Autodesk Inventor part; units mm, degrees
ref_plane "YZ Plane" through (0, 0, 0) normal (1, 0, 0) x (0, 1, 0)
ref_plane "XZ Plane" through (0, 0, 0) normal (0, 1, 0) x (-1, 0, 0)
ref_plane "XY Plane" through (0, 0, 0) normal (0, 0, 1) x (1, 0, 0)
sketch "Szkic2" plane through (0, 0, 0) normal (0, 1, 0) x (-1, 0, 0)
  line L0 (42.5, 23) -> (-42.5, 23)
  line L1 (-42.5, 23) -> (-42.5, -23)
  line L2 (-42.5, -23) -> (42.5, -23)
  line L3 (42.5, -23) -> (42.5, 23)
  line L4 (0, 91.0722) -> (0, -100.1143)
  line L5 (-78.4738, 0) -> (170.7955, 0)
  circle A0 centre (37.932, 17.8265) radius 2.25
  circle A1 centre (37.932, -17.8265) radius 2.25
  circle A2 centre (-37.932, 17.8265) radius 2.25
  circle A3 centre (-37.932, -17.8265) radius 2.25
  point P0 (0, 0)
  dimension "d7" = 46
  dimension "d8" = 85
  dimension "d14" = 4.5
  dimension "d16" = 35.653
  dimension "d18" = 23
  dimension "d21" = 75.864
  dimension "d22" = 42.5
extrude "Wyciągnięcie proste2" add sketch "Szkic2" along normal blind 2
sketch "Szkic3" plane through (0, 2, 0) normal (0, 1, 0) x (1, 0, 0)
  line L0 (-42.5, -23) -> (42.5, -23)
  line L1 (42.5, -23) -> (42.5, 23)
  line L2 (41.3, -23) -> (42.5, -23)
  line L3 (42.5, -23) -> (42.5, 23)
  line L4 (42.5, 23) -> (41.3, 23)
  line L5 (41.3, 23) -> (41.3, -23)
  line L6 (-42.5, 23) -> (-42.5, -23)
  line L7 (42.5, -23) -> (-42.5, -23)
  line L8 (-42.5, -23) -> (-42.5, -21.8)
  line L9 (-42.5, -21.8) -> (42.5, -21.8)
  line L10 (42.5, -21.8) -> (42.5, -23)
  line L11 (42.5, 23) -> (-42.5, 23)
  line L12 (-42.5, 23) -> (-42.5, 21.8)
  line L13 (-42.5, 21.8) -> (42.5, 21.8)
  line L14 (42.5, 21.8) -> (42.5, 23)
  line L15 (42.5, 23) -> (-42.5, 23)
  line L16 (-42.5, -23) -> (-41.3, -23)
  line L17 (-41.3, -23) -> (-41.3, 23)
  line L18 (-41.3, 23) -> (-42.5, 23)
  line L19 (-42.5, 23) -> (-42.5, -23)
  line L20 (42.5, -6) -> (41.3, -6)
  line L21 (41.3, -6) -> (41.3, 6)
  line L22 (41.3, 6) -> (42.5, 6)
  line L23 (36.3786, 0) -> (45.7918, 0)
  point P0 (0, 0)
  point P1 (41.3, -21.8)
  point P2 (-41.3, -21.8)
  point P3 (-41.3, 21.8)
  point P4 (41.3, 21.8)
  dimension "d25" = 1.2
  dimension "d26" = 1.2
  dimension "d27" = 1.2
  dimension "d28" = 1.2
  dimension "d29" = 12
  dimension "d30" = 6
extrude "Wyciągnięcie proste3" add sketch "Szkic3" along normal blind 10 contours L6 L9 L17 L0 | L17 L9 L5 L0 | L6 L13 L17 L9 | L5 L9 L1 L0 | L6 L11 L17 L13 | L5 L20 L1 L9 | L17 L11 L5 L13 | L13 L1 L22 L5 | L5 L4 L1 L13
sketch "Szkic5" plane through (0, 12, 0) normal (0, 1, 0) x (1, 0, 0)
  line L0 (41.3, -6) -> (41.3, -21.8)
  line L1 (42.5, -6) -> (42.5, 6)
  line L2 (41.3, -8) -> (42.5, -8)
  line L3 (42.5, -8) -> (42.5, -2)
  line L4 (42.5, -2) -> (41.3, -2)
  line L5 (41.3, -2) -> (41.3, -8)
  line L6 (34.6755, 0) -> (49.4443, 0)
  line L7 (40.0187, -6) -> (43.7777, -6)
  line L8 (41.3, 8) -> (42.5, 8)
  line L9 (42.5, 8) -> (42.5, 2)
  line L10 (42.5, 2) -> (41.3, 2)
  line L11 (41.3, 2) -> (41.3, 8)
  line L12 (40.0187, 6) -> (43.7777, 6)
  point P0 (0, 0)
  point P1 (41.3, 6)
  dimension "d33" = 6
  dimension "d34" = 2
extrude "Wyciągnięcie proste4" add sketch "Szkic5" along normal blind 1 contours L7 L3 L2 L0 | L12 L11 L8 L9
extrude "Wyciągnięcie proste5" add sketch "Szkic5" along normal mid plane 2 contours L10 L11 L12 L1 | L5 L4 L1 L7
sketch "Szkic6" plane through (42.5, 0, -23) normal (0, 0, -1) x (-1, 0, 0)
  line L0 (83.8, 12) -> (1.2, 12)
  line L1 (26, 12) -> (26, 0)
  line L2 (31.5, 12) -> (31.5, 0)
  line L3 (53.5, 12) -> (53.5, 0)
  line L4 (0, 0) -> (85, 0)
  line L5 (56.5, 12) -> (56.5, 0)
  line L6 (0, 0) -> (0, 12)
  circle A0 centre (28.6456, 7.207) radius 1.5875
  line L7 (1.2, 2) -> (83.8, 2)
  line L8 (26, 2) -> (56.5, 2)
  point P0 (42.5, 0)
  dimension "d39" = 5.5
  dimension "d40" = 22
  dimension "d41" = 3
  dimension "d42" = 31.5
  dimension "d43" = 3.175
  dimension "d55" = 5.207
sketch "Szkic8" plane through (0, 0, 0) normal (0, -1, 0) x (1, 0, 0)
  line L0 (42.5, -23) -> (-42.5, -23)
  line L1 (20.6822, -23) -> (-15.9857, -23)
  line L2 (-15.9857, -23) -> (-15.9857, -42.1071)
  line L3 (-15.9857, -42.1071) -> (20.6822, -42.1071)
  line L4 (20.6822, -42.1071) -> (20.6822, -23)
  line L5 (17, -23) -> (11, -23)
  line L6 (11, -23) -> (11, -35.8)
  line L7 (11, -35.8) -> (17, -35.8)
  line L8 (17, -35.8) -> (17, -23)
  line L9 (11, -23) -> (-11, -23)
  line L10 (-11, -23) -> (-11, -35.8)
  line L11 (-11, -35.8) -> (11, -35.8)
  line L12 (11, -35.8) -> (11, -23)
  line L13 (-11, -23) -> (-14, -23)
  line L14 (-14, -23) -> (-14, -35.8)
  line L15 (-14, -35.8) -> (-11, -35.8)
  line L16 (-11, -35.8) -> (-11, -23)
  line L17 (17, -26.8) -> (-14, -26.8)
  point P0 (0, 0)
  point P1 (11, -26.8)
  point P2 (-14, -23)
  point P3 (17, -23)
  dimension "d45" = 6
  dimension "d46" = 22
  dimension "d47" = 3
  dimension "d48" = 31.5
  dimension "d49" = 3.8
  dimension "d50" = 9
extrude "Wyciągnięcie proste6" add sketch "Szkic8" against normal blind 2 contours L6 L17 L10 L0 | L8 L7 L6 L17 | L10 L17 L14 L0 | L6 L11 L10 L17 | L10 L15 L14 L17
extrude "Wyciągnięcie proste7" add sketch "Szkic8" against normal blind 12 contours L8 L17 L6 L0
sketch "Szkic9" plane through (17, 2, -26.8) normal (0, 0, -1) x (-1, 0, 0)
  circle A0 centre (3.0287, 5.207) radius 1.4322
  line L0 (0, 0) -> (31, 0)
  point P0 (17, -2)
  dimension "d63" = 5.207
hole "Otwór2" at (13.9713, 7.207, -26.8) direction (0, 0, 1) diameter 4 depth 4 counterbore diameter 4.5 counterbore depth 0.6
properties part number "prent1"
Could you check a few things on this model? Use its own coordinates, in mm. A direction names the side the tool comes from. Coordinates: 2 decimals unless noted, no trailing zeros. Loops run counter-clockwise (first coordinate to the right, second up) from the corner with the lowest first, then second, coordinate; pieces in that order, holes last.
1. Imagine slicing it at D-D (y = 3.5). Please give me the cut outline in (x, z).
2. Imagine slicing it at B-B (z = 3.5). Please give me the cut outline in (x, y), and give its area (3 significant figures).
3. We'd pull the mould along Y, two halves only. Please class faces 1 (the face through (-1, 7, 21.8)), 2 (the face through (12.074, 8.417, -26.496)), 3 (the face through (14, 7, -22.8)), 4 (the face through (0, 12, -22)): released by +Y, released by -Y, zero draft, split by the parting line, or undercut.
4. For P1, Ø0.5, axis at x = 42, y = 12.5, coming from the -Z side; P2, Ø5, axis at x = 30, z = -7, coming from the +Y side; P3, Ø5, axis at x = 15, y = 6.5, coming from the -Z side, each with a flat end and sliding along its axis, tell me the tip position at first contact or that it passes through.
5. I need wall thicknesses on L1, parallel to X at y = 10.75, z = -6.5; L2, parallel to Z at x = 0, y = 4.5; L3, parallel to Z at x = 14.5, y = 8.75. Which ranges of each line are inside material? Lowest first, please.
6. Imagine slicing it at C-C (z = -7). Please give me the cut outline in (x, y), and give its area (3 significant figures).
7. Imagine slicing it at A-A (x = -26). Please give me the cut outline in (y, z), and give its area (3 significant figures).
8. For faces 5 (the face through (-41.3, 7, 0)), 6 (the face through (14, 4.7, -26.8)), 7 (the face through (17, 4.6, -26.6)), which set-ups out of +Z, -Z, +X, -X, +Y, -Y let a thin tool reach every point of the face, with its end or its side?
Computed values:
1. outline: (-42.5, -23) - (11, -23) - (11, -26.8) - (17, -26.8) - (17, -23) - (42.5, -23) - (42.5, -6) - (41.3, -6) - (41.3, -21.8) - (-41.3, -21.8) - (-41.3, 21.8) - (41.3, 21.8) - (41.3, 6) - (42.5, 6) - (42.5, 23) - (-42.5, 23) - close
2. outline: (-42.5, 0) - (42.5, 0) - (42.5, 2) - (-41.3, 2) - (-41.3, 12) - (-42.5, 12) - close; (41.3, 11) - (42.5, 11) - (42.5, 13) - (41.3, 13) - close
2. area: 184 mm2
3. face 1: zero draft
3. face 2: undercut
3. face 3: undercut
3. face 4: released by +Y
4. P1: stops at z = -8
4. P2: stops at y = 2
4. P3: stops at z = -26.8
5. L1: x = -42.5 to -41.3, 41.3 to 42.5
5. L2: z = -23 to -21.8, 21.8 to 23
5. L3: z = -22.8 to -21.8, 21.8 to 23
6. outline: (-42.5, 0) - (42.5, 0) - (42.5, 13) - (41.3, 13) - (41.3, 2) - (-41.3, 2) - (-41.3, 12) - (-42.5, 12) - close
6. area: 195 mm2
7. outline: (0, -23) - (12, -23) - (12, -21.8) - (2, -21.8) - (2, 21.8) - (12, 21.8) - (12, 23) - (0, 23) - close
7. area: 116 mm2
8. face 5: +Y
8. face 6: -Z, +X, -X, +Y
8. face 7: -Z, +X, +Y, -Y
